Could you check a few things on this drawing? It's one solid part, dimensions in mm from its lowest x, y, z. A direction names the side the tool comes from. Round coordinates to 2 decimals unless told otherwise and drop trailing zeros. Loops run counter-clockwise (first coordinate to the right, second up) from the corner with the lowest first, then second, coordinate; pieces in that order, holes last. Notation, with made-up numbers: M -15,39.25 L 15,39.25 A10 ccw 15,54.25 Z; hole C 79,-25.75 d9. An arc over 180 degrees is marked long. Answer as a JSON object with one key per item and string values.
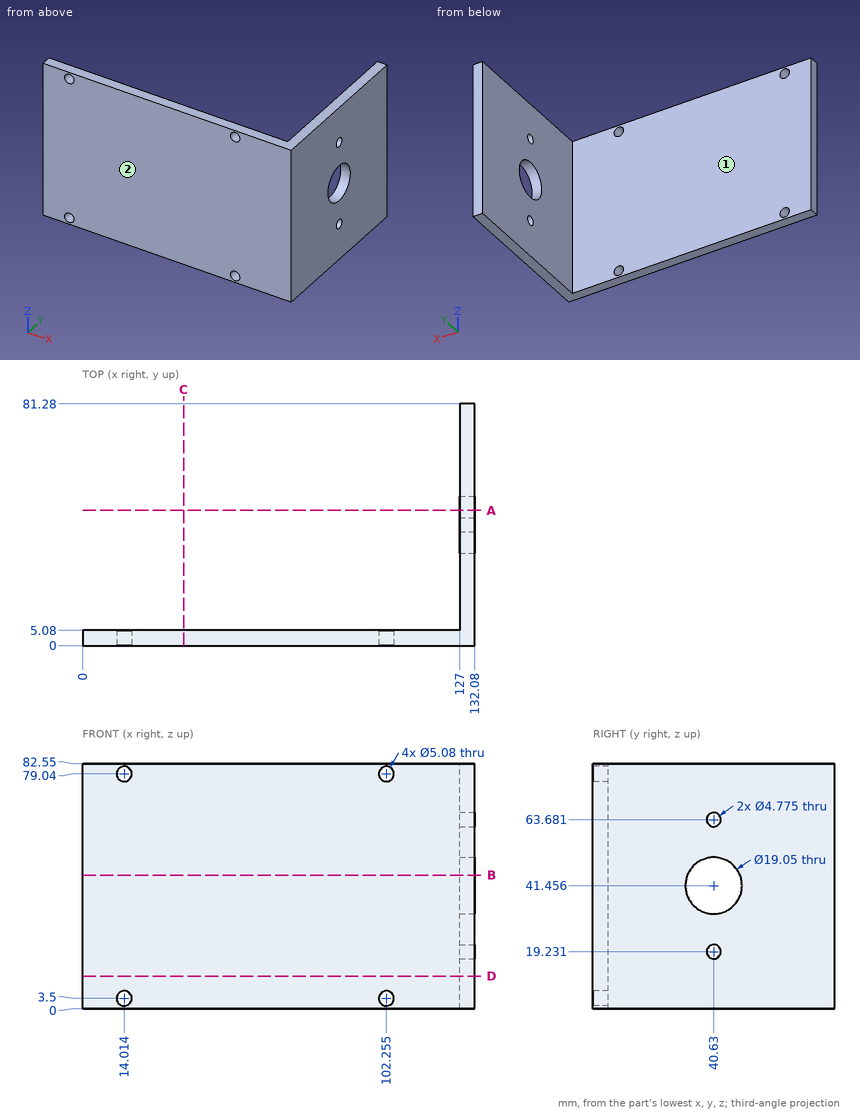
Item 1: On a 3-axis mill with a long thin cutter (end or side, diameter ignored), from which of +Z, -Z, +X, -X, +Y, -Y can I reach the whole of each face in a straight line? I mean the marked faces 1 and 2. Say none if no direction works.
Resolved:
{"face 1": "+Z, -Z, -X, +Y", "face 2": "+Z, -Z, +X, -X, -Y"}
Item 2: I want a section at C-C, the plane x = 34. Please give me the cut outline in (y, z).
Resolved:
{"outline": "M 0,0 L 5.08,0 L 5.08,82.55 L 0,82.55 Z"}
Item 3: Please list where these lines run through material, in increasing order: probe 1 along Y at (x, z) = (58.5, 14); probe 2 along X at (y, z) = (31, 71.5). Write a range as from..to.
Resolved:
{"probe 1": "0..5.08", "probe 2": "127..132.08"}
Item 4: I want a section at B-B, the plane z = 45. Please give me the cut outline in (x, y).
Resolved:
{"outline": "M 0,0 L 132.08,0 L 132.08,31.79 L 127,31.79 L 127,5.08 L 0,5.08 Z; M 127,49.47 L 132.08,49.47 L 132.08,81.28 L 127,81.28 Z"}
Item 5: I want a section at D-D, the plane z = 11. Please give me the cut outline in (x, y), then the cut area to 3 significant figures.
Resolved:
{"outline": "M 0,0 L 132.08,0 L 132.08,81.28 L 127,81.28 L 127,5.08 L 0,5.08 Z", "area": "1,060 mm²"}
Item 6: I'm going to push flat-ended pins straight in: pin 1 Ø5 at (y, z) = (51, 9.5) entering from -X; pin 2 Ø6 at (y, z) = (40.63, 19.23) entering from +X. Where does each tip first touch, or does it pass through?
Resolved:
{"pin 1": "x = 127", "pin 2": "x = 132.08"}
Item 7: I want a section at A-A, the plane y = 45.5. Please give me the cut outline in (x, z).
Resolved:
{"outline": "M 127,0 L 132.08,0 L 132.08,33.27 L 127,33.27 Z; M 127,49.64 L 132.08,49.64 L 132.08,82.55 L 127,82.55 Z"}
